```python
from build123d import *

# Parameters (mm, degrees)
F0_R     = 2
F1_DEPTH = 4
F2_DEPTH = 4
F3_DEPTH = 3


with BuildPart() as f1:
    # F0 (on Top) → F1 (new body)
    with BuildSketch(Plane.XY):
        Polygon((38.825550833, 38.3700664616), (43.825550833, 38.3700664616), (43.825550833, 43.3700664616), (43.825550833, 48.3700664616), (33.825550833, 48.3700664616), (33.825550833, 38.4970664616), (33.825550833, 38.3700664616), (34.0726979835, 38.3700664616), align=None)
        with Locations((38.825550833, 43.3700664616)):
            Circle(F0_R, mode=Mode.SUBTRACT)
        Polygon((-42.374449167, 48.3700664616), (-42.374449167, 38.3700664616), (-42.120449167, 38.3700664616), (-38.437449167, 38.3700664616), (29.888550833, 38.3700664616), (33.571550833, 38.3700664616), (33.825550833, 38.3700664616), (33.825550833, 38.4970664616), (33.825550833, 48.3700664616), align=None)
        Polygon((33.825550833, -37.5759335384), (33.825550833, -37.8299335384), (33.9456979835, -37.8299335384), (43.825550833, -37.8299335384), (43.825550833, 38.3700664616), (38.825550833, 38.3700664616), (34.0726979835, 38.3700664616), (33.825550833, 38.3700664616), (33.825550833, 38.1160664616), (33.825550833, 34.4330664616), (33.825550833, 22.7744664616), (33.825550833, 16.7800664616), (33.825550833, -1.6349335384), (33.825550833, -6.0799335384), (33.825550833, -19.9229335384), (33.825550833, -20.0499335384), (33.825550833, -33.8929335384), align=None)
        Polygon((-52.374449167, 43.3700664616), (-52.374449167, 38.3700664616), (-47.374449167, 38.3700664616), (-42.374449167, 38.3700664616), (-42.374449167, 48.3700664616), (-52.374449167, 48.3700664616), align=None)
        with Locations((-47.374449167, 43.3700664616)):
            Circle(F0_R, mode=Mode.SUBTRACT)
        Polygon((-52.374449167, 38.3700664616), (-52.374449167, -12.4299335384), (-42.374449167, -12.4299335384), (-42.374449167, 34.4330664616), (-42.374449167, 38.1160664616), (-42.374449167, 38.3700664616), (-47.374449167, 38.3700664616), align=None)
        Polygon((-52.374449167, -42.8299335384), (-52.374449167, -47.8299335384), (-47.374449167, -47.8299335384), (-42.374449167, -47.8299335384), (-42.374449167, -37.8299335384), (-52.374449167, -37.8299335384), align=None)
        with Locations((-47.374449167, -42.8299335384)):
            Circle(F0_R, mode=Mode.SUBTRACT)
        Polygon((-42.374449167, -37.8299335384), (-42.374449167, -47.8299335384), (33.825550833, -47.8299335384), (33.825550833, -37.8299335384), (33.571550833, -37.8299335384), (33.317550833, -37.8299335384), (31.285550833, -37.8299335384), (30.269550833, -37.8299335384), (29.888550833, -37.8299335384), (13.302350833, -37.8299335384), (5.885550833, -37.8299335384), (2.253350833, -37.8299335384), (-38.437449167, -37.8299335384), (-42.120449167, -37.8299335384), align=None)
        Polygon((33.825550833, -37.8299335384), (33.825550833, -47.8299335384), (38.825550833, -47.8299335384), (43.825550833, -47.8299335384), (43.825550833, -42.8299335384), (43.825550833, -37.8299335384), (33.9456979835, -37.8299335384), align=None)
        with Locations((38.825550833, -42.8299335384)):
            Circle(F0_R, mode=Mode.SUBTRACT)
    extrude(amount=F1_DEPTH)

    # F0 (on Top) → F2 (join)
    with BuildSketch(Plane.XY):
        Polygon((-52.374449167, -12.4299335384), (-52.374449167, -37.8299335384), (-42.374449167, -37.8299335384), (-42.374449167, -37.5759335384), (-42.374449167, -36.0798128688), (-42.374449167, -33.8929335384), (-42.374449167, -12.4299335384), align=None)
        Polygon((-42.374449167, -37.5759335384), (-42.374449167, -37.8299335384), (-42.120449167, -37.8299335384), (-38.437449167, -37.8299335384), (2.253350833, -37.8299335384), (5.885550833, -37.8299335384), (13.302350833, -37.8299335384), (29.888550833, -37.8299335384), (30.269550833, -37.8299335384), (31.285550833, -37.8299335384), (33.317550833, -37.8299335384), (33.571550833, -37.8299335384), (33.825550833, -37.8299335384), (33.825550833, -37.5759335384), (33.825550833, -33.8929335384), (33.825550833, -20.0499335384), (33.825550833, -19.9229335384), (33.825550833, -6.0799335384), (33.825550833, -1.6349335384), (33.825550833, 16.7800664616), (33.825550833, 22.7744664616), (33.825550833, 34.4330664616), (33.825550833, 38.1160664616), (33.825550833, 38.3700664616), (33.571550833, 38.3700664616), (29.888550833, 38.3700664616), (-38.437449167, 38.3700664616), (-42.120449167, 38.3700664616), (-42.374449167, 38.3700664616), (-42.374449167, 38.1160664616), (-42.374449167, 34.4330664616), (-42.374449167, -12.4299335384), (-42.374449167, -33.8929335384), (-42.374449167, -36.0798128688), align=None)
    extrude(amount=F2_DEPTH)

    # F0 (on Top) → F3 (cut)
    with BuildSketch(Plane.XY):
        Polygon((-42.374449167, -37.5759335384), (-42.374449167, -37.8299335384), (-42.120449167, -37.8299335384), (-38.437449167, -37.8299335384), (2.253350833, -37.8299335384), (5.885550833, -37.8299335384), (13.302350833, -37.8299335384), (29.888550833, -37.8299335384), (30.269550833, -37.8299335384), (31.285550833, -37.8299335384), (33.317550833, -37.8299335384), (33.571550833, -37.8299335384), (33.825550833, -37.8299335384), (33.825550833, -37.5759335384), (33.825550833, -33.8929335384), (33.825550833, -20.0499335384), (33.825550833, -19.9229335384), (33.825550833, -6.0799335384), (33.825550833, -1.6349335384), (33.825550833, 16.7800664616), (33.825550833, 22.7744664616), (33.825550833, 34.4330664616), (33.825550833, 38.1160664616), (33.825550833, 38.3700664616), (33.571550833, 38.3700664616), (29.888550833, 38.3700664616), (-38.437449167, 38.3700664616), (-42.120449167, 38.3700664616), (-42.374449167, 38.3700664616), (-42.374449167, 38.1160664616), (-42.374449167, 34.4330664616), (-42.374449167, -12.4299335384), (-42.374449167, -33.8929335384), (-42.374449167, -36.0798128688), align=None)
        Polygon((-52.374449167, 38.3700664616), (-52.374449167, -12.4299335384), (-42.374449167, -12.4299335384), (-42.374449167, 34.4330664616), (-42.374449167, 38.1160664616), (-42.374449167, 38.3700664616), (-47.374449167, 38.3700664616), align=None)
    extrude(amount=F3_DEPTH, mode=Mode.SUBTRACT)


solid = f1.part
```
Part model, mm, in its own coordinate system. A direction names the side the tool comes from. Round coordinates to 2 decimals unless told otherwise and drop trailing zeros. Order: outer loops, then holes, each group sorted by start corner. A loop starts at its lowest first (then second) coordinate and runs counter-clockwise, first axis right, second up. Notation, with made-up numbers: M -26.5,52.5 L 9.5,52.5 A17 ccw 9.5,80.5 Z; hole C 76.25,6.5 d7. An arc over 180 degrees is marked long. Answer in a Markdown table with one row per item. Add a question column.
Q1. Wall check: L1, parallel to Y at x = 2, z = 0.2; L2, parallel to X at y = -19.5, z = 1.1; L3, parallel to Z at x = -7, y = -16. Give the ranges that are in metal, low to high. Write a range as from..to.
Q2. Cut at C-C on z = 0.7. Give the cut face in (x, y), and give its area (3 significant figures).
Q3. Cut at B-B on y = -31. Give the cut face in (x, z), and give its area (3 significant figures).
Q4. Cut at D-D on y = -7. Give the cut face in (x, z).
Q5. Pin check, flat tip, straight feed: pin 1 (10 mm diameter, centred on x = 17.5, y = 5.5, fed in from -Z). Stop position of the tip, or through.
Q6. Mould opens along X. For faces 4 (the face through (33.826, 0, 1)), 5 (the face through (-5, -47.83, 2)), 6 (the face through (-52.374, -9.7, 3.3)), 7 (the face through (-45.467, 43.971, 1.972)) say: +X half, -X half, draft (parallel to the pull), parting line (faces both ways), or undercut.
Q7. 3-axis set-ups, long thin cutter, end or side, ignore diameter. For faces 1 (the face through (-47, -12.43, 1)), 2 (the face through (-5, -37.83, 1)), 3 (the face through (39.748, -44.604, 1.972)): which of +Z, -Z, +X, -X, +Y, -Y reach the whole face in a straight line?
Q8. Cut at A-A on x = -44. Give the cut face in (y, z).
Established:
| question | item | result |
|---|---|---|
| 1 | L1 | y = -47.83..-37.83, 38.37..48.37 |
| 1 | L2 | x = -52.37..-42.37, 33.83..43.83 |
| 1 | L3 | z = 3..4 |
| 2 | outline | M -52.37,-47.83 L 43.83,-47.83 L 43.83,48.37 L -52.37,48.37 L -52.37,38.37 L 33.83,38.37 L 33.83,-37.83 L -42.37,-37.83 L -42.37,-12.43 L -52.37,-12.43 Z; hole C -47.37,-42.83 d4; hole C -47.37,43.37 d4; hole C 38.83,-42.83 d4; hole C 38.83,43.37 d4 |
| 2 | area | 2,890 mm2 |
| 3 | outline | M -52.37,0 L -42.37,0 L -42.37,3 L 33.83,3 L 33.83,0 L 43.83,0 L 43.83,4 L -52.37,4 Z |
| 3 | area | 156 mm2 |
| 4 | outline | M -52.37,3 L 33.83,3 L 33.83,0 L 43.83,0 L 43.83,4 L -52.37,4 Z |
| 5 | pin 1 | stops at z = 3 |
| 6 | face 4 | undercut |
| 6 | face 5 | draft |
| 6 | face 6 | -X half |
| 6 | face 7 | undercut |
| 7 | face 1 | -Z, -X |
| 7 | face 2 | -Z |
| 7 | face 3 | +Z, -Z |
| 8 | outline | M -47.83,0 L -12.43,0 L -12.43,3 L 38.37,3 L 38.37,0 L 48.37,0 L 48.37,4 L -47.83,4 Z |
